Input: part model. Units: mm. Frame: model coordinates. A direction names the side the tool comes from. Round coordinates to 2 decimals unless told otherwise and drop trailing zeros. Loops run counter-clockwise (first coordinate to the right, second up) from the corner with the lowest first, then second, coordinate; pieces in that order, holes last. Notation, with made-up numbers: (35, -4.5) -> (85, -4.5) arc R28 ccw to (85, 34.5) -> close; hole circle Ø4 at (34.25, 69). An arc over 180 degrees is marked (long way). Answer as a JSON object with one key per item and string values. Group by question number.
Item 1: Section query B-B on x = 0. Return loops of the section in (y, z).
Item 2: Material intervals for line 1 (Y direction, x = 0, z = 6.75); line 2 (Y direction, x = 0, z = 3.75); line 3 (Y direction, x = 2.5, z = 1.25), sorted ascending. Write a range as [from, to].
Item 3: Section query A-A on z = 7. Return loops of the section in (x, y).
Item 4: Section query D-D on x = 6. Return loops of the section in (y, z), and give its area (3 significant figures).
Item 5: Section query C-C on y = 2.75. Return loops of the section in (x, z), and give its area (3 significant figures).
Item 6: Draft query along Y for faces 3 (the cylindrical face through (-0.35, 8.44, 4.93)), 4 (the flat face through (-7, -13, 5)), 5 (the flat face through (10, 0, 5)), 6 (the flat face through (-7, 13, 5)). Return one class per face: released by +Y, released by -Y, zero draft, split by the parting line, or undercut.
Item 7: Set-up query: faces 1 (the flat face through (4, -3, 10)), 2 (the flat face through (0, -6.45, 3)). Return all of +Z, -Z, +X, -X, +Y, -Y with unobstructed straight access to the full face (end or side cutting, diameter ignored); none if empty.
Item 8: Pin query (flat end, axial travel): pin 1 (3 mm diameter, centred on x = 2.5, y = -1, fed in from +Z). Return the tip coordinate at first contact, or that it passes through.
from build123d import *

# Parameters (mm, degrees)
SKETCH_1_W      = 20
SKETCH_1_H      = 30
SKETCH_1_R      = 1.6
EXTRUDE_1_DEPTH = 10
CHAMFER_1_SIZE  = 5
SKETCH_2_W      = 15
SKETCH_2_H      = 15
SKETCH_2_R      = 4.75
EXTRUDE_2_DEPTH = 3.8


with BuildPart() as part:
    # 草圖1 → 填料-伸長1 (new body)
    with BuildSketch(Plane.XY):
        Rectangle(SKETCH_1_W, SKETCH_1_H)
        with Locations((0, 10)):
            Circle(SKETCH_1_R, mode=Mode.SUBTRACT)
        with Locations((0, -10)):
            Circle(SKETCH_1_R, mode=Mode.SUBTRACT)
        Polygon((7.447818473, 0), (3.723909236, 6.45), (-3.723909236, 6.45), (-7.447818473, 0), (-3.723909236, -6.45), (3.723909236, -6.45), align=None, mode=Mode.SUBTRACT)
    extrude(amount=EXTRUDE_1_DEPTH)

    # 導角1
    chamfer_1_edges = [part.edges().sort_by_distance(p)[0] for p in [
        (10, -15, 5),
        (-10, -15, 5),
        (-10, 15, 5),
        (10, 15, 5),
    ]]
    chamfer(chamfer_1_edges, length=CHAMFER_1_SIZE)

    # 草圖2 → 填料-伸長2 (add)
    with BuildSketch(Plane.XY.offset(10)):
        Rectangle(SKETCH_2_W, SKETCH_2_H)
        Circle(SKETCH_2_R, mode=Mode.SUBTRACT)
    extrude(amount=-EXTRUDE_2_DEPTH)


solid = part.part
Solved:
{
 "1": {"outline": "(-15, 0) -> (-11.6, 0) -> (-11.6, 10) -> (-15, 10) -> close; (-8.4, 0) -> (-6.45, 0) -> (-6.45, 6.2) -> (-4.75, 6.2) -> (-4.75, 10) -> (-8.4, 10) -> close; (4.75, 6.2) -> (6.45, 6.2) -> (6.45, 0) -> (8.4, 0) -> (8.4, 10) -> (4.75, 10) -> close; (11.6, 0) -> (15, 0) -> (15, 10) -> (11.6, 10) -> close"},
 "2": {"line 1": "[-15, -11.6], [-8.4, -4.75], [4.75, 8.4], [11.6, 15]", "line 2": "[-15, -11.6], [-8.4, -6.45], [6.45, 8.4], [11.6, 15]", "line 3": "[-15, -6.45], [6.45, 15]"},
 "3": {"outline": "(-10, -10) -> (-5, -15) -> (5, -15) -> (10, -10) -> (10, 10) -> (5, 15) -> (-5, 15) -> (-10, 10) -> close; hole circle Ø9.5 at (0, 0); hole circle Ø3.2 at (0, -10); hole circle Ø3.2 at (0, 10)"},
 "4": {"outline": "(-14, 0) -> (-2.51, 0) -> (-2.51, 6.2) -> (2.51, 6.2) -> (2.51, 0) -> (14, 0) -> (14, 10) -> (-14, 10) -> close", "area": "249 mm²"},
 "5": {"outline": "(-10, 0) -> (-5.86, 0) -> (-5.86, 6.2) -> (-3.87, 6.2) -> (-3.87, 10) -> (-10, 10) -> close; (3.87, 6.2) -> (5.86, 6.2) -> (5.86, 0) -> (10, 0) -> (10, 10) -> (3.87, 10) -> close", "area": "97.9 mm²"},
 "6": {"face 3": "undercut", "face 4": "released by -Y", "face 5": "zero draft", "face 6": "released by +Y"},
 "7": {"face 1": "+Z, +X, -X, +Y, -Y", "face 2": "-Z"},
 "8": {"pin 1": "through"}
}
